Autodesk Inventor part; units mm, degrees
ref_plane "YZ Plane" through (0, 0, 0) normal (1, 0, 0) x (0, 1, 0)
ref_plane "XZ Plane" through (0, 0, 0) normal (0, 1, 0) x (-1, 0, 0)
ref_plane "XY Plane" through (0, 0, 0) normal (0, 0, 1) x (1, 0, 0)
sketch "Sketch1" plane through (0, 0, 0) normal (0, 1, 0) x (-1, 0, 0)
  circle A0 centre (0, 0) radius 12.7
  dimension "d0" = 25.4
extrude "Extrusion1" add sketch "Sketch1" along normal blind 1.5748
sketch "Sketch2" plane through (0, 0, 0) normal (0, -1, 0) x (1, 0, 0)
  circle A0 centre (0, 0) radius 9.271
  line L0 (0, -9.271) -> (0, -7.271)
  line L1 (9.271, 0) -> (8.271, 0)
  line L2 (8.271, 0) -> (7.771, 0)
  line L3 (7.771, 0) -> (6.771, 0)
  line L4 (6.771, 0) -> (6.271, 0)
  line L5 (6.271, 0) -> (5.271, 0)
  line L6 (5.271, 0) -> (4.771, 0)
  line L7 (4.771, 0) -> (3.771, 0)
  line L8 (3.771, 0) -> (3.271, 0)
  line L9 (3.271, 0) -> (2.271, 0)
  line L10 (2.271, 0) -> (1.771, 0)
  line L11 (1.771, 0) -> (0.771, 0)
  line L12 (0.771, 0) -> (0.271, 0)
  line L13 (0, 9.271) -> (0, 7.271)
  arc A1 (0, -9.271) -> (0, 9.271) centre (-158.4465, 0) ccw
  arc A2 (0, -9.271) -> (0, 9.271) centre (-55.3547, 0) ccw
  arc A3 (0, -9.271) -> (0, 9.271) centre (-23.3809, 0) ccw
  arc A4 (0, -9.271) -> (0, 9.271) centre (-17.7882, 0) ccw
  arc A5 (0, -9.271) -> (0, 9.271) centre (-11.5029, 0) ccw
  arc A6 (0, -9.271) -> (0, 9.271) centre (-9.5109, 0) ccw
  arc A7 (0, -9.271) -> (0, 9.271) centre (-6.6222, 0) ccw
  arc A8 (0, -9.271) -> (0, 9.271) centre (-5.5177, 0) ccw
  arc A9 (0, -9.271) -> (0, 9.271) centre (-3.7176, 0) ccw
  arc A10 (0, -9.271) -> (0, 9.271) centre (-2.9615, 0) ccw
  arc A11 (0, -9.271) -> (0, 9.271) centre (-1.6448, 0) ccw
  arc A12 (0, -9.271) -> (0, 9.271) centre (-1.0605, 0) ccw
  circle A13 centre (0, 9.271) radius 1
  circle A14 centre (0, -9.271) radius 1
  point P0 (0.974, -9.0443)
  point P1 (0.986, -9.1043)
  point P2 (0.986, 9.1043)
  point P3 (0.974, 9.0443)
  point P4 (0.9357, 8.9182)
  point P5 (0.9084, 8.8528)
  point P6 (0.9084, -8.8528)
  point P7 (0.9357, -8.9182)
  point P8 (0.7874, -8.6546)
  point P9 (0.8347, -8.7203)
  point P10 (0.8347, 8.7203)
  point P11 (0.7874, 8.6546)
  point P12 (0.6008, -8.4716)
  point P13 (0.6706, -8.5292)
  point P14 (0.6706, 8.5292)
  point P15 (0.6008, 8.4716)
  point P16 (0.4399, 8.373)
  point P17 (0.35, 8.3343)
  point P18 (0.35, -8.3343)
  point P19 (0.4399, -8.373)
  point P20 (0.0553, -8.2725)
  point P21 (0.1564, -8.2833)
  point P22 (0.1564, 8.2833)
  point P23 (0.0553, 8.2725)
  dimension "d3" = 18.542
  dimension "d4" = 2
  dimension "d5" = 1
  dimension "d6" = 0.5
  dimension "d7" = 1
  dimension "d8" = 0.5
  dimension "d9" = 1
  dimension "d10" = 0.5
  dimension "d11" = 1
  dimension "d12" = 0.5
  dimension "d13" = 1
  dimension "d14" = 0.5
  dimension "d15" = 1
  dimension "d16" = 0.5
  dimension "d17" = 2
  dimension "d18" = 2
  dimension "d19" = 2
extrude "Extrusion2" add sketch "Sketch2" along normal blind 1.8 contours A12 A14 A11 L2 | L2 A11 A13 A12 | A13 A2 L12 A1 | A13 A4 L10 A3 | A13 A6 L8 A5 | A13 A8 L6 A7 | A13 A10 L4 A9 | A1 L12 A2 A14 | A3 L10 A4 A14 | A5 L8 A6 A14 | A7 L6 A8 A14 | A9 L4 A10 A14
mirror "Mirror1" about plane through (0, 0, 0) normal (1, 0, 0) of "Extrusion2"
properties part number "flow director r1"
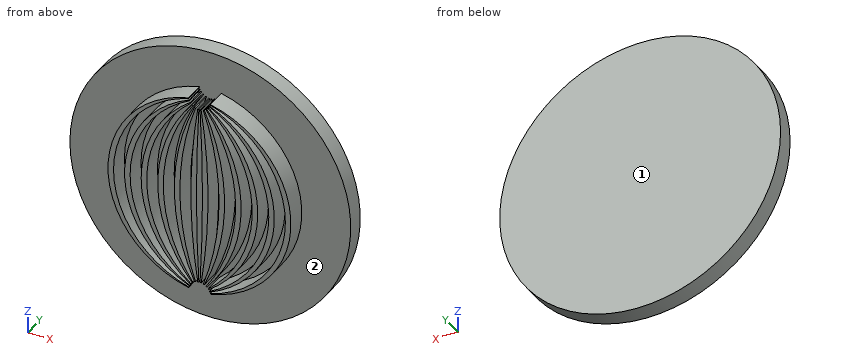
Input: part model. Units: mm. Frame: model coordinates. Face numbers are marked on the shaded views. Give positions to 0.01 mm unless a question says otherwise; leave off trailing zeros. Loops run counter-clockwise (first coordinate to the right, second up) from the corner with the lowest first, then second, coordinate; pieces in that order, holes last. Notation, with made-up numbers: M 38.25,79 L 43.25,79 A15 ccw 43.25,101 Z; hole C -18,33.5 d6. An arc over 180 degrees is marked long. Use CSV: the item, a comma, the result in double quotes.
(1) Section B-B, the plane x = -4.25. Return loops of the section in (y, z).
Outcome:
outline,"M -1.8,-7.67 L 0,-7.67 L 0,-11.97 L 1.57,-11.97 L 1.57,11.97 L 0,11.97 L 0,7.67 L -1.8,7.67 L -1.8,7.34 L 0,7.34 L 0,6.54 L -1.8,6.54 L -1.8,6.02 L 0,6.02 L 0,4.58 L -1.8,4.58 L -1.8,3.41 L 0,3.41 L 0,-3.41 L -1.8,-3.41 L -1.8,-4.58 L 0,-4.58 L 0,-6.02 L -1.8,-6.02 L -1.8,-6.54 L 0,-6.54 L 0,-7.34 L -1.8,-7.34 Z"
(2) Section C-C, the plane z = 9.5. Return loops of the section in (x, y), plus the area to 3 significant figures.
Outcome:
outline,"M -8.43,0 L 8.43,0 L 8.43,1.57 L -8.43,1.57 Z"
area,"26.5 mm²"
(3) Pull-direction query (X, two-part tool) for the marked faces 1 and 2; classes: pulls with the +X half, pulls with the -X half, needs draft (parallel to the pull), parting line crosses it, or undercut.
Outcome:
face 1,"needs draft"
face 2,"undercut"
(4) Pin query (flat end, axial travel): P1, Ø2, axis at x = -4.5, z = -10, coming from the -Y side; P2, Ø2, axis at x = 1.5, y = 1, coming from the +Z side; P3, Ø1.5, axis at x = 7.5, y = 0, coming from the -Z side. Return the tip coordinate at first contact, or that it passes through.
Outcome:
P1,"stops at y = 0"
P2,"stops at z = 12.69"
P3,"stops at z = -10.76"
(5) Material intervals for L1, parallel to Y at x = 0, z = -3.5; L2, parallel to X at y = 0.6, z = 4.5; L3, parallel to Z at x = -7, y = -0.9, sorted ascending. Write a range as [from, to].
Outcome:
L1,"y = [0, 1.57]"
L2,"x = [-11.88, 11.88]"
L3,"z = [-4.7, -3.73], [3.73, 4.7]"
(6) Section A-A, the plane y = -0.55. Count the separate pieces of the cut face and the enclosed holes in it, plus the area to 3 significant figures.
Outcome:
separate pieces,"12"
enclosed holes,"0"
area,"84.7 mm²"
